Build history of the part. All positions in model axes, mm. Round coordinates to 2 decimals unless told otherwise and drop trailing zeros. Loops run counter-clockwise (first coordinate to the right, second up) from the corner with the lowest first, then second, coordinate; pieces in that order, holes last.
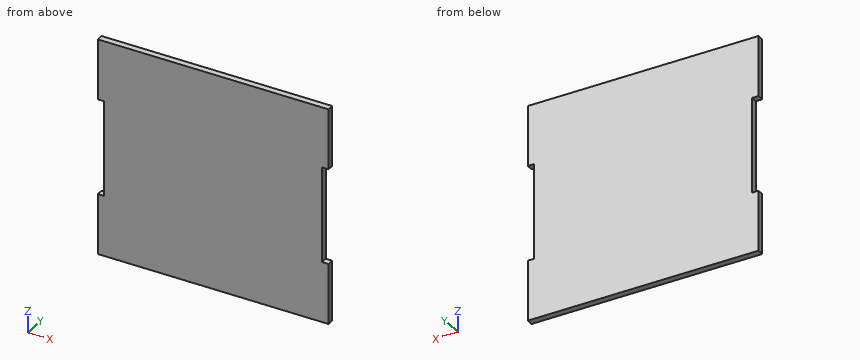
Autodesk Inventor part; units mm, degrees
ref_plane "YZ Plane" through (0, 0, 0) normal (1, 0, 0) x (0, 1, 0)
ref_plane "XZ Plane" through (0, 0, 0) normal (0, 1, 0) x (-1, 0, 0)
ref_plane "XY Plane" through (0, 0, 0) normal (0, 0, 1) x (1, 0, 0)
sketch "Sketch1" plane through (0, 0, 0) normal (0, 1, 0) x (-1, 0, 0)
  line L0 (90, 85) -> (-90, 85)
  line L1 (-90, 85) -> (-90, -85)
  line L2 (-90, -85) -> (90, -85)
  line L3 (90, -85) -> (90, 85)
  line L4 (90, 85) -> (-90, -85) construction
  line L5 (-90, 85) -> (90, -85) construction
  point P0 (0, 0)
  dimension "d0" = 170
  dimension "d1" = 180
extrude "Extrusion1" add sketch "Sketch1" along normal blind 5
sketch "Sketch2" plane through (0, 5, 0) normal (0, 1, 0) x (1, 0, 0)
  line L0 (85, 37.5) -> (95, 37.5)
  line L1 (95, 37.5) -> (95, -37.5)
  line L2 (95, -37.5) -> (85, -37.5)
  line L3 (85, -37.5) -> (85, 37.5)
  line L4 (90, -85) -> (90, 85)
  line L5 (85, 37.5) -> (95, -37.5) construction
  line L6 (95, 37.5) -> (85, -37.5) construction
  line L7 (0, 0) -> (0, 85) construction
  line L8 (90, 85) -> (-90, 85)
  line L9 (-85, 37.5) -> (-95, 37.5)
  line L10 (-95, 37.5) -> (-95, -37.5)
  line L11 (-95, -37.5) -> (-85, -37.5)
  line L12 (-85, -37.5) -> (-85, 37.5)
  line L13 (-90, -85) -> (-90, 85)
  line L14 (-85, 37.5) -> (-95, -37.5) construction
  line L15 (-95, 37.5) -> (-85, -37.5) construction
  point P0 (90, 0)
  point P1 (-90, 0)
  dimension "d4" = 75
  dimension "d5" = 5
extrude "Extrusion2" cut sketch "Sketch2" against normal blind 10
properties part number "Gel base"
(1) Pin check, flat tip, straight feed: P1, Ø2.5, axis at y = 2, z = 17.5, coming from the -X side. Stop position of the tip, or through.
Responses:
P1: stops at x = -85
(2) Slice it at A-A on y = 2.3. List the corners of the cut face in (x, z), plus the area to 4 significant figures.
Responses:
outline: (-90, -85) - (90, -85) - (90, -37.5) - (85, -37.5) - (85, 37.5) - (90, 37.5) - (90, 85) - (-90, 85) - (-90, 37.5) - (-85, 37.5) - (-85, -37.5) - (-90, -37.5) - close
area: 29,850 mm2
(3) Probe line 1 (X direction, y = 1.15, z = -13.5). List the from-to ranges inside material, lowest first.
Responses:
line 1: x = -85 to 85
(4) Slice it at B-B on z = 11.5. List the corners of the cut face in (x, y), plus the area to 3 significant figures.
Responses:
outline: (-85, 0) - (85, 0) - (85, 5) - (-85, 5) - close
area: 850 mm2
